from build123d import *

# Parameters (mm, degrees)
F0_R           = 6
F1_DEPTH       = 29
F3_D           = 4.2
F3_DEPTH       = 14.4
F3_CBORE_D     = 9.75
F3_CBORE_DEPTH = 5
F3_TIP         = 1.2618073


with BuildPart() as f1:
    # F0 (on Front) → F1 (new body)
    with BuildSketch(Plane.XZ):
        Circle(F0_R)
    extrude(amount=F1_DEPTH)

    # F3
    with Locations(Plane.XZ.offset(29)):
        with Locations((0, 0)):
            CounterBoreHole(F3_D / 2, F3_CBORE_D / 2, F3_CBORE_DEPTH, depth=F3_DEPTH)
            with Locations((0, 0, -(F3_DEPTH + F3_TIP / 2))):  # 118° drill point
                Cone(0, F3_D / 2, F3_TIP, mode=Mode.SUBTRACT)


solid = f1.part
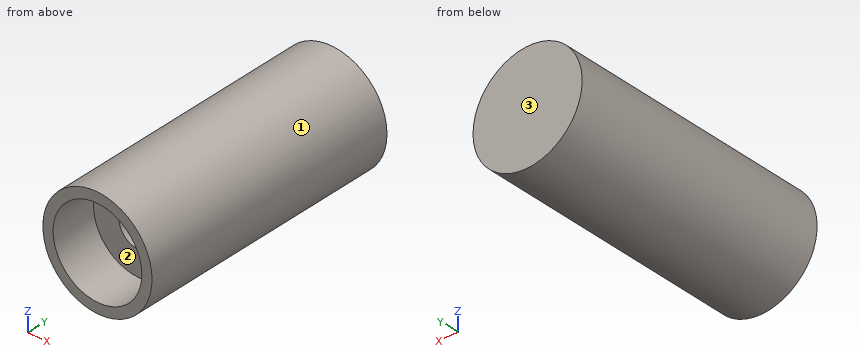
The model under review builds one solid part; all positions refer to its coordinate system, in mm. Face numbers are marked on the shaded views. Round coordinates to 2 decimals unless told otherwise and drop trailing zeros. Loops run counter-clockwise (first coordinate to the right, second up) from the corner with the lowest first, then second, coordinate; pieces in that order, holes last. Notation, with made-up numbers: (79.5, 50.5) -> (128.5, 50.5) arc R25 cw to (128.5, 85.5) -> close; hole circle Ø4 at (-6.5, 36.25). An arc over 180 degrees is marked (long way). Write item = value, one per line. Start each with the question number.
Item 1: Take a section at D-D on y = -11.25. Give the boundary of the cut face in (x, z), plus the area to 3 significant figures.
Item 2: Take a section at B-B on z = 2.5. Give the boundary of the cut face in (x, y), plus the area to 3 significant figures.
Item 3: Mouldability with a two-part tool opening along Z and no side actions: class the marked faces 1, 2 and 3 as released by +Z, released by -Z, zero draft, split by the parting line, or undercut.
Item 4: Take a section at C-C on y = -21.5. Give the boundary of the cut face in (x, z), plus the area to 3 significant figures.
Item 5: Take a section at A-A on x = 3. Give the boundary of the cut face in (y, z).
Item 6: To check wall thickness, follow L1, parallel to Z at x = 0, y = -25.45 (3 decimals); L2, parallel to Z at x = 0, y = -19.75; L3, parallel to Y at x = 2, z = -2. State the ranges of each line that lie inside material, in increasing order.
Item 7: Insertion check: pin 1 (2 mm diameter, centred on x = -2, y = -14, fed in from -Z); pin 2 (5 mm diameter, centred on x = 0, z = 0, fed in from -Y); pin 3 (1.5 mm diameter, centred on y = -6.5, z = 1.5, fed in from -X). Each pin has a flat end and moves straight along its axis. Give the tip position at first contact, or say it passes through.
Result:
q1.outline = circle Ø12 at (0, 0)
q1.area = 113 mm²
q2.outline = (-5.45, -29) -> (-4.19, -29) -> (-4.19, -24) -> (4.19, -24) -> (4.19, -29) -> (5.45, -29) -> (5.45, 0) -> (-5.45, 0) -> close
q2.area = 275 mm²
q3.face_1 = split by the parting line
q3.face_2 = undercut
q3.face_3 = zero draft
q4.outline = circle Ø12 at (0, 0); hole circle Ø4.2 at (0, 0)
q4.area = 99.2 mm²
q5.outline = (-29, -5.2) -> (0, -5.2) -> (0, 5.2) -> (-29, 5.2) -> (-29, 3.84) -> (-24, 3.84) -> (-24, -3.84) -> (-29, -3.84) -> close
q6.L1 = -6 to -4.875, 4.875 to 6
q6.L2 = -6 to -2.1, 2.1 to 6
q6.L3 = -24 to 0
q7.pin_1 = -5.92
q7.pin_2 = -24
q7.pin_3 = -5.95
